```python
from build123d import *

# Parameters (mm, degrees)
F0_R     = 3.75
F1_DEPTH = 3
F2_R     = 1.4
F3_DEPTH = 6.096


# Not quite as in the source:
# - a feature names something its author has since deleted; it is built from what else it names


with BuildPart() as f1:
    # F0 (on Top) → F1 (new body)
    with BuildSketch(Plane.XY):
        with BuildLine():
            ThreePointArc((-3.1727983399, 6.7958333333), (0, 4.25), (3.1727983399, 6.7958333333))
            ThreePointArc((3.1727983399, 6.7958333333), (0, 7.5), (-3.1727983399, 6.7958333333))
        make_face()
        with BuildLine():
            Line((11.0098453548, 3.1369193284), (3.1727983399, 6.7958333333))
            ThreePointArc((3.1727983399, 6.7958333333), (5.8592267319, 4.6818225195), (7.3284005906, 1.5951629335))
            ThreePointArc((7.3284005906, 1.5951629335), (8.9045755783, 2.9977340645), (11.0098453548, 3.1369193284))
        make_face()
        with BuildLine():
            ThreePointArc((7.3284005906, 1.5951629335), (5.8592267319, 4.6818225195), (3.1727983399, 6.7958333333))
            ThreePointArc((3.1727983399, 6.7958333333), (0, 4.25), (-3.1727983399, 6.7958333333))
            ThreePointArc((-3.1727983399, 6.7958333333), (-5.8592267319, 4.6818225195), (-7.3284005906, 1.5951629335))
            ThreePointArc((-7.3284005906, 1.5951629335), (-7.0163398656, 0.8245610709), (-6.91, 0))
            ThreePointArc((-6.91, 0), (-7.0163398656, -0.8245610709), (-7.3284005906, -1.5951629335))
            ThreePointArc((-7.3284005906, -1.5951629335), (-5.9282154859, -4.5941551076), (-3.3735330862, -6.6984531435))
            ThreePointArc((-3.3735330862, -6.6984531435), (-3.2735278386, -6.7478897064), (-3.1727983399, -6.7958333333))
            ThreePointArc((-3.1727983399, -6.7958333333), (0, -4.25), (3.1727983399, -6.7958333333))
            ThreePointArc((3.1727983399, -6.7958333333), (5.8592267319, -4.6818225195), (7.3284005906, -1.5951629335))
            ThreePointArc((7.3284005906, -1.5951629335), (6.91, 0), (7.3284005906, 1.5951629335))
        make_face()
        Circle(F0_R, mode=Mode.SUBTRACT)
        with BuildLine():
            ThreePointArc((-3.1727983399, 6.7958333333), (0, 7.5), (3.1727983399, 6.7958333333))
            ThreePointArc((3.1727983399, 6.7958333333), (3.2306419335, 7.1458069768), (3.25, 7.5))
            ThreePointArc((3.25, 7.5), (-0.3541930232, 10.7306419335), (-3.1727983399, 6.7958333333))
        make_face()
        with BuildLine():
            ThreePointArc((-7.3284005906, 1.5951629335), (-5.8592267319, 4.6818225195), (-3.1727983399, 6.7958333333))
            Line((-3.1727983399, 6.7958333333), (-11.0098453548, 3.1369193284))
            ThreePointArc((-11.0098453548, 3.1369193284), (-8.9045755783, 2.9977340645), (-7.3284005906, 1.5951629335))
        make_face()
        with BuildLine():
            ThreePointArc((11.0098453548, 3.1369193284), (8.9045755783, 2.9977340645), (7.3284005906, 1.5951629335))
            ThreePointArc((7.3284005906, 1.5951629335), (7.4569767476, 0.8021831371), (7.5, 0))
            ThreePointArc((7.5, 0), (7.4569767476, -0.8021831371), (7.3284005906, -1.5951629335))
            ThreePointArc((7.3284005906, -1.5951629335), (8.9045755783, -2.9977340645), (11.0098453548, -3.1369193284))
            ThreePointArc((11.0098453548, -3.1369193284), (12.7411332204, -1.9749053898), (13.41, 0))
            ThreePointArc((13.41, 0), (12.7411332204, 1.9749053898), (11.0098453548, 3.1369193284))
        make_face()
        with BuildLine():
            ThreePointArc((7.5, 0), (7.4569767476, 0.8021831371), (7.3284005906, 1.5951629335))
            ThreePointArc((7.3284005906, 1.5951629335), (6.91, 0), (7.3284005906, -1.5951629335))
            ThreePointArc((7.3284005906, -1.5951629335), (7.4569767476, -0.8021831371), (7.5, 0))
        make_face()
        with BuildLine():
            ThreePointArc((-6.91, 0), (-7.0163398656, 0.8245610709), (-7.3284005906, 1.5951629335))
            ThreePointArc((-7.3284005906, 1.5951629335), (-7.5, 0), (-7.3284005906, -1.5951629335))
            ThreePointArc((-7.3284005906, -1.5951629335), (-7.0163398656, -0.8245610709), (-6.91, 0))
        make_face()
        with BuildLine():
            ThreePointArc((-7.3284005906, -1.5951629335), (-7.5, 0), (-7.3284005906, 1.5951629335))
            ThreePointArc((-7.3284005906, 1.5951629335), (-8.9045755783, 2.9977340645), (-11.0098453548, 3.1369193284))
            ThreePointArc((-11.0098453548, 3.1369193284), (-13.3855431521, -0.3979590107), (-10.2219168602, -3.2494101468))
            ThreePointArc((-10.2219168602, -3.2494101468), (-8.5469535603, -2.8214501915), (-7.3284005906, -1.5951629335))
        make_face()
        with BuildLine():
            ThreePointArc((11.0098453548, -3.1369193284), (8.9045755783, -2.9977340645), (7.3284005906, -1.5951629335))
            ThreePointArc((7.3284005906, -1.5951629335), (5.8592267319, -4.6818225195), (3.1727983399, -6.7958333333))
            Line((3.1727983399, -6.7958333333), (11.0098453548, -3.1369193284))
        make_face()
        with BuildLine():
            ThreePointArc((-3.3735330862, -6.6984531435), (-5.9282154859, -4.5941551076), (-7.3284005906, -1.5951629335))
            ThreePointArc((-7.3284005906, -1.5951629335), (-8.5469535603, -2.8214501915), (-10.2219168602, -3.2494101468))
            Line((-10.2219168602, -3.2494101468), (-3.3735330862, -6.6984531435))
        make_face()
        with BuildLine():
            ThreePointArc((3.25, -7.5), (3.2306419335, -7.1458069768), (3.1727983399, -6.7958333333))
            ThreePointArc((3.1727983399, -6.7958333333), (0, -7.5), (-3.1727983399, -6.7958333333))
            ThreePointArc((-3.1727983399, -6.7958333333), (-3.1731688138, -6.7975046766), (-3.1735384072, -6.7991762148))
            ThreePointArc((-3.1735384072, -6.7991762148), (-0.3524912598, -10.7308280536), (3.25, -7.5))
        make_face()
        with BuildLine():
            ThreePointArc((-3.1727983399, -6.7958333333), (0, -7.5), (3.1727983399, -6.7958333333))
            ThreePointArc((3.1727983399, -6.7958333333), (0, -4.25), (-3.1727983399, -6.7958333333))
        make_face()
    extrude(amount=F1_DEPTH)

    # F2 (on face) → F3 (cut)
    with BuildSketch(Plane.XY.offset(3)):
        with Locations((-9.25, 0)):
            Circle(F2_R)
        with Locations((9.25, 0)):
            Circle(F2_R)
    extrude(amount=-F3_DEPTH, mode=Mode.SUBTRACT)


solid = f1.part
```
Verification items for the finished model (mm, model axes). Round coordinates to 2 decimals unless told otherwise and drop trailing zeros. Write each loop counter-clockwise with the first axis right and the second up, starting at its lowest first coordinate (ties: lowest second). Pieces come first, ordered by that corner, then holes. Notation, with made-up numbers: (57, 83.25) - (90, 83.25) arc R24 ccw to (90, 119.25) - close; hole circle Ø1 at (37, 79.25). An arc over 180 degrees is marked (long way). Answer as a JSON object with one key per item and string values. Group by question number.
Q1. Section check C-C, the plane x = -9.25. Enter the section's corners in (y, z).
Q2. Section check B-B, the plane x = 0. Enter the section's corners in (y, z), plus the area to 3 significant figures.
Q3. Section check D-D, the plane y = 9. Enter the section's corners in (x, z), plus the area to 3 significant figures.
Q4. Section check A-A, the plane z = 2.15. Give the number of separate pieces and of enclosed holes in the cut face, plus the area to 3 significant figures.
Q5. Go/stop test with a flat-tipped pin: pin 1 Ø1 at (y, z) = (3.5, 1) entering from -X. Record where the tip stops, or that it passes through.
Q6. Thickness scan on line 1 (Y direction, x = 0, z = 2); line 2 (Y direction, x = 9.25, z = 2.35); line 3 (X direction, y = -3, z = 1.2). Record the ranges inside material, lowest first.
Q7. Mould release check, pull along Y, two halves, no side actions. Record for faces 1 (the flat face through (-6.846, -4.95, 1.479)), 2 (the cylindrical face through (-3.746, 0.165, 1.479)), 3 (the flat face through (-3, 3, 0)): released by +Y, released by -Y, zero draft, split by the parting line, or undercut.
Found:
{
 "1": {"outline": "(-3.74, 0) - (-1.4, 0) - (-1.4, 3) - (-3.74, 3) - close; (1.4, 0) - (3.96, 0) - (3.96, 3) - (1.4, 3) - close"},
 "2": {"outline": "(-10.75, 0) - (-3.75, 0) - (-3.75, 3) - (-10.75, 3) - close; (3.75, 0) - (10.75, 0) - (10.75, 3) - (3.75, 3) - close", "area": "42.0 mm^2"},
 "3": {"outline": "(-2.88, 0) - (2.88, 0) - (2.88, 3) - (-2.88, 3) - close", "area": "17.3 mm^2"},
 "4": {"separate pieces": "1", "enclosed holes": "3", "area": "249 mm^2"},
 "5": {"pin 1": "stops at x = -11.41"},
 "6": {"line 1": "y = -10.75 to -3.75, 3.75 to 10.75", "line 2": "y = -3.96 to -1.4, 1.4 to 3.96", "line 3": "x = -11.41 to -2.25, 2.25 to 11.41"},
 "7": {"face 1": "released by -Y", "face 2": "undercut", "face 3": "zero draft"}
}
